Geometry check sheet. Reference: the model listing, model coordinates, mm. Face numbers are marked on the shaded views. Give positions to 0.01 mm unless a question says otherwise; leave off trailing zeros. Write each loop counter-clockwise with the first axis right and the second up, starting at its lowest first coordinate (ties: lowest second). Pieces come first, ordered by that corner, then holes. Notation, with made-up numbers: M 13.25,13.5 L 61.25,13.5 A10 ccw 61.25,28.5 Z; hole C 18.25,-4 d7. An arc over 180 degrees is marked long. Write each question's results on one line, items separated by ' | '.
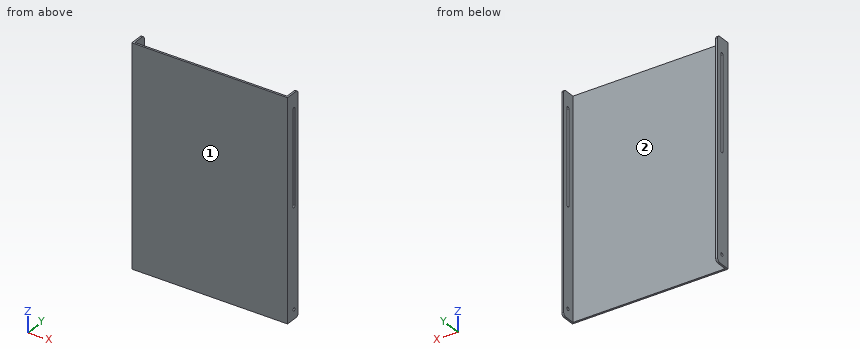
```python
from build123d import *

# Parameters (mm, degrees)
EXTRUDE_THIN1_DEPTH     = 350
CUT_EXTRUDE1_DEPTH      = 613.372435696
CUT_EXTRUDE1_DEPTH_BACK = 613.372435696
SKETCH2_R               = 5
FILLET1_R               = 10


with BuildPart() as part:
    # Sketch1 → Extrude-Thin1 (new, symmetric)
    with BuildSketch(Plane.XY):
        Polygon((-250, 50), (-250, 0), (250, 0), (250, 50), (244, 50), (244, 6), (-244, 6), (-244, 50), align=None)
    extrude(amount=EXTRUDE_THIN1_DEPTH, both=True)

    # Sketch2 → Cut-Extrude1 (cut, two sides: drawn at the far end of the back side and taken through both)
    with BuildSketch(Plane(origin=(250, 0, 0), x_dir=(0, 0, -1), z_dir=(1, 0, 0)).offset(-CUT_EXTRUDE1_DEPTH_BACK)):
        with Locations((320, 30)):
            Circle(SKETCH2_R)
        with BuildLine():
            Line((-300, 35), (0, 35))
            ThreePointArc((0, 35), (5, 30), (0, 25))
            Line((0, 25), (-300, 25))
            ThreePointArc((-300, 25), (-305, 30), (-300, 35))
        make_face()
    extrude(amount=CUT_EXTRUDE1_DEPTH + CUT_EXTRUDE1_DEPTH_BACK, mode=Mode.SUBTRACT)

    # Fillet1
    fillet1_edges = [part.edges().sort_by_distance(p)[0] for p in [
        (247, 50, 350),
        (247, 50, -350),
        (-247, 50, 350),
        (-247, 50, -350),
    ]]
    fillet(fillet1_edges, radius=FILLET1_R)


solid = part.part
```
Q1. Section check C-C (z = -295). Enter the section's corners in (x, y).
Answer key:
outline: M -250,0 L 250,0 L 250,50 L 244,50 L 244,6 L -244,6 L -244,50 L -250,50 Z
Q2. Section check D-D (x = -69). Enter the section's corners in (y, z), then the cut area to 3 significant figures.
Answer key:
outline: M 0,-350 L 6,-350 L 6,350 L 0,350 Z | area: 4,200 mm2
Q3. Depth check by flat-ended pin: P1, Ø5, axis at y = 31, z = 252, coming from the +X side; P2, Ø2, axis at x = 47.5, z = -243, coming from the +Y side. Enter the tip coordinate at first touch or a pass-through.
Answer key:
P1: passes through | P2: stops at y = 6
Q4. Section check A-A (z = 268.5). Enter the section's corners in (x, y).
Answer key:
outline: M -250,0 L 250,0 L 250,25 L 244,25 L 244,6 L -244,6 L -244,25 L -250,25 Z; M -250,35 L -244,35 L -244,50 L -250,50 Z; M 244,35 L 250,35 L 250,50 L 244,50 Z
Q5. Material ranges on probe 1 along Z at (x, y) = (247.5, 30); probe 2 along X at (y, z) = (33, -184); probe 3 along Y at (x, z) = (-246.85, -320), recorded low to high. Write a range as [from, to].
Answer key:
probe 1: z = [-350, -325], [-315, -5], [305, 350] | probe 2: x = [-250, -244], [244, 250] | probe 3: y = [0, 25], [35, 50]
Q6. Release check for a two-part mould opening along X. For the marked faces 1 and 2 record: released by +X, released by -X, zero draft, split by the parting line, or undercut.
Answer key:
face 1: zero draft | face 2: undercut
Q7. Section check B-B (y = 15). Enter the section's corners in (x, z), then the cut area to 3 significant figures.
Answer key:
outline: M -250,-350 L -244,-350 L -244,350 L -250,350 Z; M 244,-350 L 250,-350 L 250,350 L 244,350 Z | area: 8,400 mm2
